Work out the finished part from the listing and answer in its coordinate system (mm). A direction names the side the tool comes from. Coordinates: 2 decimals unless noted, no trailing zeros. Order: outer loops, then holes, each group sorted by start corner. A loop starts at its lowest first (then second) coordinate and runs counter-clockwise, first axis right, second up.
1. Determine the mould class of faces 4 (the flat face through (-1.3, 18, -1.3)), 5 (the cylindrical face through (0, 7, -2)), 6 (the flat face through (0.76, 17.014, -1.293)) for opening direction Z: +Z half, -Z half, draft (parallel to the pull), parting line (faces both ways), or undercut.
2. The part is cut by section B-B, the plane z = 0. Give the vertices of the cut face in (x, y), then the cut area to 3 significant figures.
3. Flat-ended cylindrical pins translate along their axes: pin 1 Ø2 at (x, y) = (1, 12) entering from +Z; pin 2 Ø4 at (y, z) = (9.5, 1.5) entering from -X; pin 3 Ø2 at (y, z) = (16, 2) entering from +X. Find the tip coordinate at first contact, or state that the pin passes through.
4. A tool of negligible diameter and unlimited length cuts with its end or side. For faces 1 (the flat face through (0, 0, 0)), 2 (the flat face through (-2, 14, -2)), 3 (the flat face through (1.5, 17, 0)), from which of +Z, -Z, +X, -X, +Y, -Y can it reach the whole face along a straight path? Write none if from no direction.
5. The part is cut by section C-C, the plane y = 2.5. Give the vertices of the cut face in (x, z).
6. Find the intervals of material crossed by probe 1 along Y at (x, z) = (0.75, -1.25); probe 2 along Y at (x, z) = (2, 1.5); probe 3 along X at (y, z) = (2.5, -1), in increasing order.
7. The part is cut by section A-A, the plane y = 16.75. Give the vertices of the cut face in (x, z).
Autodesk Inventor part; units mm, degrees
ref_plane "anf_ge_1_XY" through (0, 14, 0) normal (0, 1, 0) x (1, 0, 0)
ref_plane "anf_ge_1_YZ" through (0, 14, 0) normal (1, 0, 0) x (0, 0, -1)
ref_plane "anf_ge_1_ZX" through (0, 14, 0) normal (0, 0, -1) x (0, 1, 0)
sketch "Skizze_1" plane through (0, 0, 0) normal (0, 0, 1) x (1, 0, 0)
  line L0 (0, 18) -> (0, 0)
  line L1 (0, 0) -> (-1.5705, 0)
  line L2 (-1.5705, 0) -> (-2, 0.4295)
  line L3 (-2, 0.4295) -> (-2, 14)
  line L4 (-2, 14) -> (-3.5, 14)
  line L5 (-3.5, 14) -> (-3.5, 17.6)
  arc A0 (-3.1, 18) -> (-3.5, 17.6) centre (-3.1, 17.6) ccw
  line L6 (-3.1, 18) -> (0, 18)
  line L7 (0, 18) -> (0, 0)
revolve "Revolution1" add sketch "Skizze_1" angle 360 about axis through (0, 18, 0) along (0, 1, 0)
thread "Thread1"
sketch "Skizze_2" plane through (0, 18, 0) normal (0, 1, 0) x (-1, 0, 0)
  line L0 (-1.5, -0.866) -> (0, -1.7321)
  line L1 (0, -1.7321) -> (1.5, -0.866)
  line L2 (1.5, -0.866) -> (1.5, 0.866)
  line L3 (1.5, 0.866) -> (0, 1.7321)
  line L4 (0, 1.7321) -> (-1.5, 0.866)
  line L5 (-1.5, 0.866) -> (-1.5, -0.866)
extrude "Extrusion1" cut sketch "Skizze_2" against normal blind 2
ref_plane "anf_ge_1_XY" through (0, 14, 0) normal (0, 1, 0) x (1, 0, 0)
ref_plane "anf_ge_1_YZ" through (0, 14, 0) normal (1, 0, 0) x (0, 0, -1)
ref_plane "anf_ge_1_ZX" through (0, 14, 0) normal (0, 0, -1) x (0, 1, 0)
properties part number "62311400GA_2" material "Steel AISI 1045 225 ANLD"
Geometry says:
1. face 4: draft
1. face 5: parting line
1. face 6: undercut
2. outline: (-3.5, 14) - (-2, 14) - (-2, 0.43) - (-1.57, 0) - (1.57, 0) - (2, 0.43) - (2, 14) - (3.5, 14) - (3.5, 17.6) arc R0.4 ccw to (3.1, 18) - (1.5, 18) - (1.5, 16) - (-1.5, 16) - (-1.5, 18) - (-3.1, 18) arc R0.4 ccw to (-3.5, 17.6) - close
2. area: 77.7 mm2
3. pin 1: stops at z = 2
3. pin 2: stops at x = -2
3. pin 3: stops at x = 3.35
4. face 1: +Z, -Z, +X, -X, -Y
4. face 2: -Y
4. face 3: +Y
5. outline: circle Ø4 at (0, 0)
6. probe 1: y = 0 to 16
6. probe 2: y = 14 to 18
6. probe 3: x = -1.73 to 1.73
7. outline: circle Ø7 at (0, 0); hole (-1.5, -0.87) - (0, -1.73) - (1.5, -0.87) - (1.5, 0.87) - (0, 1.73) - (-1.5, 0.87) - close
